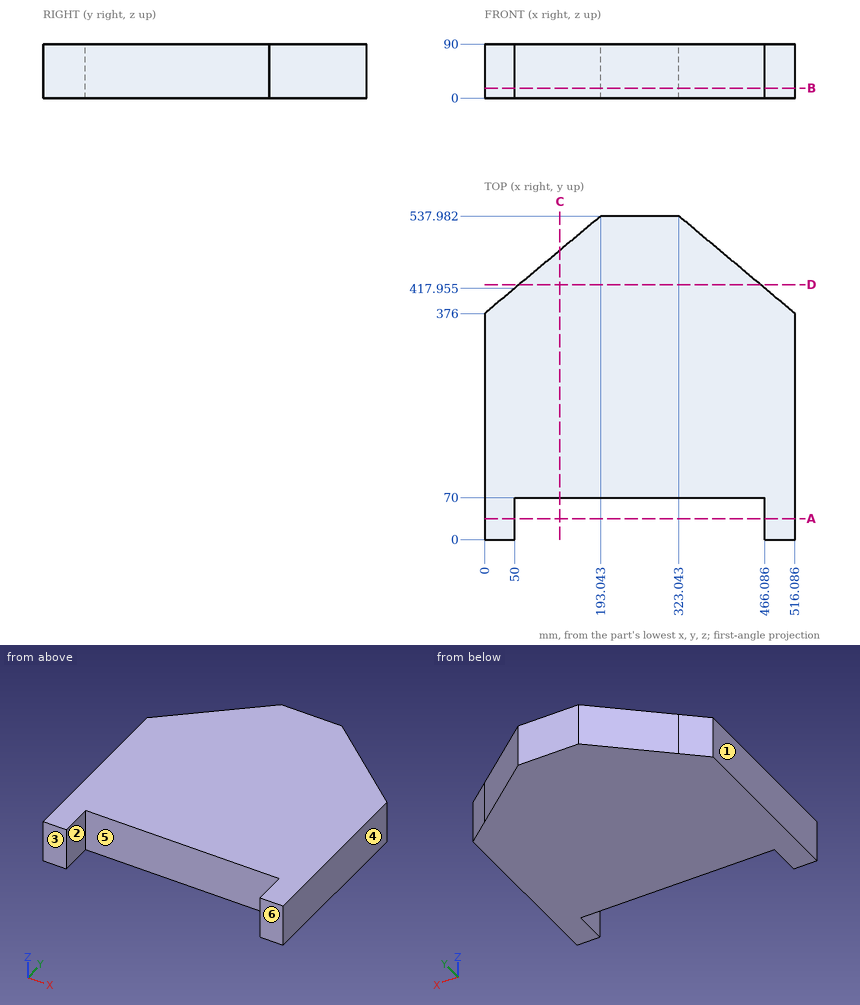
For this review, use the dimensioned drawing (mm, ordinates from the lowest corner) and the shaded views. A direction names the side the tool comes from. Give positions to 0.01 mm unless a question says otherwise; leave off trailing zeros. Loops run counter-clockwise (first coordinate to the right, second up) from the corner with the lowest first, then second, coordinate; pieces in that order, holes last. Notation, with made-up numbers: (28, 82.25) -> (33, 82.25) arc R15 cw to (33, 99.25) -> close; hole circle Ø8 at (46.25, 28.25). An arc over 180 degrees is marked (long way). One line per question, with ' | ' between items. Start each with the question number.
(1) We need section A-A (y = 35). State the section outline as (x, z) points, and give its area (3 significant figures).
(2) We need section D-D (y = 424). State the section outline as (x, z) points (1 decimal), and give its area (4 significant figures).
(3) Insertion check: P1, Ø4, axis at x = 392.5, z = 21, coming from the +Y side. The pin has a flat end and moves straight along its axis. Give the tip position at first contact, or say it passes through.
(4) We need section B-B (z = 16.5). State the section outline as (x, y) points (1 decimal).
(5) Draft analysis for pull direction X (two halves, no side actions). For the marked faces 1, 2, 3 and 4, state which applies: +X half, -X half, draft (parallel to the pull), parting line (faces both ways), or undercut.
(6) We need section C-C (x = 125). State the section outline as (y, z) points.
(7) For line 1 (X direction, y = 58.5, z = 54.5); line 2 (Y direction, x = 288.5, z = 63); line 3 (Y direction, x = 139, z = 47) (1 decimal), list the stretches that pass through material, from the lowest coordinate up.
(8) For the marked faces 5 and 6, list the 3-axis set-ups (+Z, -Z, +X, -X, +Y, -Y) from which the entire face can be reached by the end or side of a thin tool; tool diameter is ignored.
The answers:
1) outline: (0, 0) -> (50, 0) -> (50, 90) -> (0, 90) -> close; (466.09, 0) -> (516.09, 0) -> (516.09, 90) -> (466.09, 90) -> close | area: 9,000 mm^2
2) outline: (57.2, 0) -> (458.9, 0) -> (458.9, 90) -> (57.2, 90) -> close | area: 36,150 mm^2
3) P1: stops at y = 481.38
4) outline: (0, 0) -> (50, 0) -> (50, 70) -> (466.1, 70) -> (466.1, 0) -> (516.1, 0) -> (516.1, 376) -> (323, 538) -> (193, 538) -> (0, 376) -> close
5) face 1: -X half | face 2: undercut | face 3: draft | face 4: +X half
6) outline: (70, 0) -> (480.89, 0) -> (480.89, 90) -> (70, 90) -> close
7) line 1: x = 0 to 50, 466.09 to 516.09 | line 2: y = 70 to 537.98 | line 3: y = 70 to 492.6
8) face 5: +Z, -Z, -Y | face 6: +Z, -Z, +X, -X, -Y
